Geometry check sheet. Reference: the model listing, model coordinates, mm. Face numbers are marked on the shaded views. Give positions to 0.01 mm unless a question says otherwise; leave off trailing zeros. Write each loop counter-clockwise with the first axis right and the second up, starting at its lowest first coordinate (ties: lowest second). Pieces come first, ordered by that corner, then holes. Notation, with made-up numbers: (83.5, 75.5) - (115.5, 75.5) arc R19 ccw to (115.5, 112.5) - close; hole circle Ø11 at (41, 54.25). An arc over 180 degrees is marked (long way). Use a Markdown table: item, result.
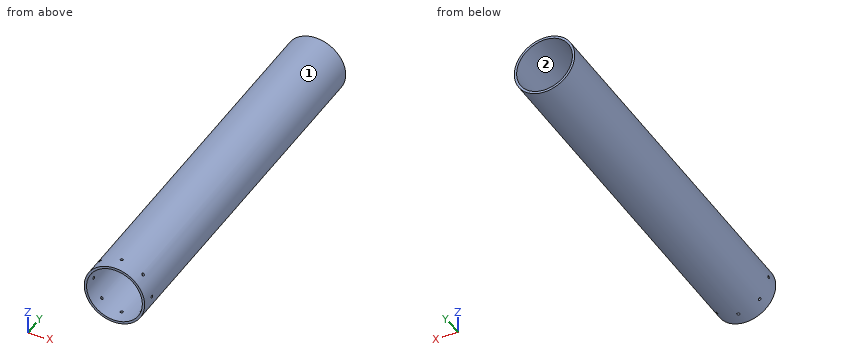
```python
from build123d import *

# Parameters (mm, degrees)
SKETCH1_R           = 40
SKETCH1_R_2         = 36.95
BOSS_EXTRUDE1_DEPTH = 500
SKETCH2_R           = 1.9
CUT_EXTRUDE1_DEPTH  = 66
CIRPATTERN2_COUNT   = 8


with BuildPart() as part:
    # Sketch1 → Boss-Extrude1 (new body)
    with BuildSketch(Plane(origin=(0, 0, 0), x_dir=(1, 0, 0), z_dir=(0, 1, 0))):
        Circle(SKETCH1_R)
        Circle(SKETCH1_R_2, mode=Mode.SUBTRACT)
    extrude(amount=BOSS_EXTRUDE1_DEPTH)

    # Sketch2 → Cut-Extrude1 (cut)
    with BuildSketch(Plane.XY):
        with Locations((0, 18)):
            Circle(SKETCH2_R)
    cut_extrude1 = extrude(amount=-CUT_EXTRUDE1_DEPTH, mode=Mode.SUBTRACT)

    # CirPattern2: Cut-Extrude1 ×8 about axis
    cirpattern2_axis = Axis((0, 500, 0), (0, -1, 0))
    for i in range(1, CIRPATTERN2_COUNT):
        add(cut_extrude1.rotate(cirpattern2_axis, i * 360 / CIRPATTERN2_COUNT), mode=Mode.SUBTRACT)


solid = part.part
```
1) Section check B-B on y = 465.5. Record the boundary of the cut face in (x, z).
Working result:
| item | result |
|---|---|
| outline | circle Ø80 at (0, 0); hole circle Ø73.9 at (0, 0) |
2) Mould release check, pull along Z, two halves, no side actions. Record for the marked faces 1 and 2: pulls with the +Z half, pulls with the -Z half, needs draft (parallel to the pull), parting line crosses it, or undercut.
Working result:
| item | result |
|---|---|
| face 1 | parting line crosses it |
| face 2 | undercut |
3) Section check A-A on z = 19.5. Record the boundary of the cut face in (x, y).
Working result:
| item | result |
|---|---|
| outline | (-34.92, 0) - (-31.39, 0) - (-31.39, 500) - (-34.92, 500) - close; (31.39, 0) - (34.92, 0) - (34.92, 500) - (31.39, 500) - close |
4) Material ranges on L1, parallel to Z at x = 0, y = 363; L2, parallel to Y at x = -37.95, z = 0, recorded low to high. Write a range as from..to.
Working result:
| item | result |
|---|---|
| L1 | z = -40..-36.95, 36.95..40 |
| L2 | y = 0..16.1, 19.9..500 |
5) Section check C-C on x = 10. Record the boundary of the cut face in (y, z), then the cut area to 3 significant figures.
Working result:
| item | result |
|---|---|
| outline | (0, -38.73) - (500, -38.73) - (500, -35.57) - (0, -35.57) - close; (0, 35.57) - (500, 35.57) - (500, 38.73) - (0, 38.73) - close |
| area | 3,160 mm² |
6) Depth check by flat-ended pin: P1, Ø2, axis at x = -24.5, y = 157, coming from the +Z side; P2, Ø1.5, axis at x = -12.5, y = 234.5, coming from the +Z side. Enter the tip coordinate at first touch or a pass-through.
Working result:
| item | result |
|---|---|
| P1 | stops at z = 32.37 |
| P2 | stops at z = 38.24 |
